```python
from build123d import *

# Parameters (mm, degrees)
F0_W           = 81.1
F0_H           = 66.25
F1_DEPTH       = 5.6
F3_D           = 3.45
F4_D           = 2.39
F6_D           = 3.7973
F6_CSINK_D     = 7.7978
F6_CSINK_ANGLE = 82
F8_DEPTH       = 3.9998
F7_W           = 34.1
F7_H           = 8.5
F7_W_2         = 14.45
F7_H_2         = 11
F7_W_3         = 11
F7_H_3         = 7
F7_H_4         = 4.125
F9_DEPTH       = 5.6
F10_R          = 2


with BuildPart() as f1:
    # F0 (on Top) → F1 (new body)
    with BuildSketch(Plane.XY):
        Rectangle(F0_W, F0_H)
    extrude(amount=F1_DEPTH)

    # F3 (through all)
    with Locations(Plane.XY.offset(5.6)):
        with Locations((-27.6, 12.75), (27.6, 28.75), (-27.6, -8), (27.6, 8), (27.6, -12.75), (-27.6, -28.75)):
            Hole(F3_D / 2)

    # F4 (through all)
    with Locations(Plane.XY.offset(5.6)):
        with Locations((-35.88, 8), (35.88, 12.75), (35.88, -28.75)):
            Hole(F4_D / 2)

    # F6 (through all)
    with Locations(Plane.XY.offset(5.6)):
        with Locations((0, 0), (-9.779, 0), (9.779, 0), (19.05, 0), (-19.05, 0)):
            CounterSinkHole(F6_D / 2, F6_CSINK_D / 2, counter_sink_angle=F6_CSINK_ANGLE)

    # F7 (on face) → F8 (cut, through all)
    with BuildSketch(Plane.XY):
        Polygon((-38.55, -5.5), (-38.55, -31.125), (-19.05, -31.125), (-19.05, -25), (-33.5, -25), (-33.5, -16.5), (-19.05, -16.5), (-19.05, -5.5), align=None)
        Polygon((-38.55, 31.125), (-38.55, 5.5), (-19.05, 5.5), (-19.05, 16.5), (-33.5, 16.5), (-33.5, 25), (-19.05, 25), (-19.05, 31.125), align=None)
        Polygon((19.05, 16.5), (19.05, 5.5), (38.55, 5.5), (38.55, 31.125), (19.05, 31.125), (19.05, 25), (33.5, 25), (33.5, 16.5), align=None)
        Polygon((19.05, -25), (19.05, -31.125), (38.55, -31.125), (38.55, -5.5), (19.05, -5.5), (19.05, -16.5), (33.5, -16.5), (33.5, -25), align=None)
    extrude(amount=F8_DEPTH, mode=Mode.SUBTRACT)

    # F7 (on face) → F9 (cut, through all)
    with BuildSketch(Plane.XY):
        with Locations((0, -20.75)):
            Rectangle(F7_W, F7_H)
        with Locations((0, 20.75)):
            Rectangle(F7_W, F7_H)
        with Locations((-26.275, -20.75)):
            Rectangle(F7_W_2, F7_H)
        with Locations((26.275, -20.75)):
            Rectangle(F7_W_2, F7_H)
        with Locations((26.275, 20.75)):
            Rectangle(F7_W_2, F7_H)
        with Locations((-26.275, 20.75)):
            Rectangle(F7_W_2, F7_H)
        with Locations((0, 11)):
            Rectangle(F7_W, F7_H_2)
        with Locations((0, -11)):
            Rectangle(F7_W, F7_H_2)
        with Locations((-31.05, 0)):
            Rectangle(F7_W_3, F7_H_3)
        with Locations((31.05, 0)):
            Rectangle(F7_W_3, F7_H_3)
        with Locations((0, 27.0625)):
            Rectangle(F7_W, F7_H_4)
        with Locations((0, -27.0625)):
            Rectangle(F7_W, F7_H_4)
    extrude(amount=F9_DEPTH, mode=Mode.SUBTRACT)

    # F10
    f10_edges = [f1.edges().sort_by_distance(p)[0] for p in [
        (-40.55, 33.125, 2.8),
        (40.55, 33.125, 2.8),
        (40.55, -33.125, 2.8),
        (-40.55, -33.125, 2.8),
        (-17.05, 5.5, 2.8),
        (17.05, 5.5, 2.8),
        (-17.05, -5.5, 2.8),
        (17.05, -5.5, 2.8),
        (38.55, 31.125, 1.9999),
        (38.55, -31.125, 1.9999),
        (-38.55, 31.125, 1.9999),
        (-38.55, -31.125, 1.9999),
        (-17.05, 29.125, 2.8),
        (17.05, 29.125, 2.8),
        (17.05, -29.125, 2.8),
        (-17.05, -29.125, 2.8),
    ]]
    fillet(f10_edges, radius=F10_R)


solid = f1.part
```
Build history of the part. All positions in model axes, mm. A direction names the side the tool comes from. Give positions to 0.01 mm unless a question says otherwise; leave off trailing zeros. Loops run counter-clockwise (first coordinate to the right, second up) from the corner with the lowest first, then second, coordinate; pieces in that order, holes last. Notation, with made-up numbers: (27.5, 32) -> (58.5, 32) arc R27 cw to (58.5, 68) -> close; hole circle Ø8 at (35.5, -38). An arc over 180 degrees is marked (long way). One line per question, with ' | ' between items. Start each with the question number.
1) 3-axis set-ups, long thin cutter, end or side, ignore diameter. For faces 1 (the flat face through (19.05, -18, 2)), 2 (the flat face through (0, 5.5, 3)): which of +Z, -Z, +X, -X, +Y, -Y reach the whole face in a straight line?
2) Cut at B-B (x = 0). Give the cut face in (y, z) (3 decimals), plus the area to 3 significant figures.
3) Cut at D-D (x = 27.6). Count the separate pieces of the cut face and the enclosed holes in it, plus the area to 3 significant figures.
4) Two-plate mould, pull along X, no slides. Class faces 3 (the flat face through (-40.55, 0, 3)), 4 (the flat face through (-1, -33.125, 3)), 5 (the flat face through (29, 5.5, 2)), 6 (the flat face through (31, 3.5, 3)): released by +X, released by -X, zero draft, split by the parting line, or undercut.
5) Probe L1, parallel to X at y = 24, z = 2.8; L2, parallel to Y at x = 13, z = 1.7 (3 decimals); L3, parallel to X at y = -3, z = 1.8. List the from-to ranges inside material, lowest first.
6) Pin check, flat tips, straight feed: pin 1 (4.5 mm diameter, centred on x = 27.6, y = 28.75, fed in from -Z); pin 2 (3.5 mm diameter, centred on x = 9.779, y = 0, fed in from +Z). Stop position of each tip, or through.
7) Cut at C-C (y = -23). Give the cut face in (x, z), plus the area to 3 significant figures.
8) Cut at A-A (y = -12.75). Give the cut face in (x, z) (3 decimals).
Return value:
1) face 1: -Z | face 2: +Z, -Z
2) outline: (-33.125, 0) -> (-29.125, 0) -> (-29.125, 5.6) -> (-33.125, 5.6) -> close; (-5.5, 0) -> (-1.899, 0) -> (-1.899, 3.299) -> (-3.899, 5.6) -> (-5.5, 5.6) -> close; (1.899, 0) -> (5.5, 0) -> (5.5, 5.6) -> (3.899, 5.6) -> (1.899, 3.299) -> close; (29.125, 0) -> (33.125, 0) -> (33.125, 5.6) -> (29.125, 5.6) -> close | area: 80.5 mm^2
3) separate pieces: 7 | enclosed holes: 0 | area: 83.0 mm^2
4) face 3: released by -X | face 4: zero draft | face 5: undercut | face 6: undercut
5) L1: -40.55 to -38.55, -19.05 to -17.05, 17.05 to 19.05, 38.55 to 40.55 | L2: -33.125 to -29.125, -5.5 to 5.5, 29.125 to 33.125 | L3: -40.55 to -36.55, -25.55 to 25.55, 36.55 to 40.55
6) pin 1: z = 4 | pin 2: through
7) outline: (-40.55, 0) -> (-38.55, 0) -> (-38.55, 4) -> (-33.5, 4) -> (-33.5, 5.6) -> (-40.55, 5.6) -> close; (-19.05, 0) -> (-17.05, 0) -> (-17.05, 5.6) -> (-19.05, 5.6) -> close; (17.05, 0) -> (19.05, 0) -> (19.05, 5.6) -> (17.05, 5.6) -> close; (33.5, 4) -> (38.55, 4) -> (38.55, 0) -> (40.55, 0) -> (40.55, 5.6) -> (33.5, 5.6) -> close | area: 61.0 mm^2
8) outline: (-40.55, 0) -> (-38.55, 0) -> (-38.55, 4) -> (-19.05, 4) -> (-19.05, 0) -> (-17.05, 0) -> (-17.05, 5.6) -> (-40.55, 5.6) -> close; (17.05, 0) -> (19.05, 0) -> (19.05, 4) -> (25.875, 4) -> (25.875, 5.6) -> (17.05, 5.6) -> close; (29.325, 4) -> (38.55, 4) -> (38.55, 0) -> (40.55, 0) -> (40.55, 5.6) -> (29.325, 5.6) -> close
